Autodesk Inventor part; units mm, degrees
ref_plane "YZ Plane" through (0, 0, 0) normal (1, 0, 0) x (0, 1, 0)
ref_plane "XZ Plane" through (0, 0, 0) normal (0, 1, 0) x (-1, 0, 0)
ref_plane "XY Plane" through (0, 0, 0) normal (0, 0, 1) x (1, 0, 0)
sketch "Sketch1" plane through (0, 0, 0) normal (0, 0, 1) x (1, 0, 0)
  line L0 (-25.4, 63.5) -> (25.4, 63.5)
  line L1 (38.1, 50.8) -> (38.1, -50.8)
  line L2 (25.4, -63.5) -> (-25.4, -63.5)
  line L3 (-38.1, -50.8) -> (-38.1, 50.8)
  line L4 (-38.1, 63.5) -> (38.1, -63.5) construction
  line L5 (38.1, 63.5) -> (-38.1, -63.5) construction
  arc A0 (-25.4, 63.5) -> (-38.1, 50.8) centre (-25.4, 50.8) ccw
  arc A1 (38.1, 50.8) -> (25.4, 63.5) centre (25.4, 50.8) ccw
  arc A2 (25.4, -63.5) -> (38.1, -50.8) centre (25.4, -50.8) ccw
  arc A3 (-38.1, -50.8) -> (-25.4, -63.5) centre (-25.4, -50.8) ccw
  line L6 (25.4, 69.85) -> (-25.4, 69.85)
  arc A4 (-25.4, 69.85) -> (-44.45, 50.8) centre (-25.4, 50.8) ccw
  line L7 (-44.45, 50.8) -> (-44.45, -50.8)
  arc A5 (-44.45, -50.8) -> (-25.4, -69.85) centre (-25.4, -50.8) ccw
  line L8 (-25.4, -69.85) -> (25.4, -69.85)
  arc A6 (25.4, -69.85) -> (44.45, -50.8) centre (25.4, -50.8) ccw
  line L9 (44.45, -50.8) -> (44.45, 50.8)
  arc A7 (44.45, 50.8) -> (25.4, 69.85) centre (25.4, 50.8) ccw
  point P0 (0, 0)
  dimension "d0" = 127
  dimension "d1" = 76.2
  dimension "d2" = 12.7
  dimension "d3" = 6.35
extrude "Extrusion1" add sketch "Sketch1" against normal blind 127
properties part number "class1" material "Iron, Ductile"
Build history of the part. All positions in model axes, mm. A direction names the side the tool comes from. Round coordinates to 2 decimals unless told otherwise and drop trailing zeros. Write each loop counter-clockwise with the first axis right and the second up, starting at its lowest first coordinate (ties: lowest second). Pieces come first, ordered by that corner, then holes.
1) Drill centre lines: probe 1 along Y at (x, z) = (-15.5, -71); probe 2 along X at (y, z) = (6, -114); probe 3 along X at (y, z) = (56, -6.5). Where is each one in solid material? Low to high.
2) 3-axis set-ups, long thin cutter, end or side, ignore diameter. For faces 5 (the flat face through (0, -63.5, -63)), 6 (the flat face through (-40, 6, -127)): which of +Z, -Z, +X, -X, +Y, -Y reach the whole face in a straight line?
3) Pin check, flat tip, straight feed: pin 1 (2 mm diameter, centred on x = -35.5, z = -69, fed in from -Y). Stop position of the tip, or through.
4) Mould opens along X. For faces 1 (the flat face through (0, 69.85, -63)), 2 (the flat face through (-44.45, 1, -63)), 3 (the flat face through (38.1, 1, -63)), 4 (the cylindrical face through (39.02, 64.12, -62.61)) say: +X half, -X half, draft (parallel to the pull), parting line (faces both ways), or undercut.
5) Band-saw the part on A-A, the plane y = -48.5. List the corners of the cut face in (x, z).
6) Band-saw the part on C-C, the plane z = -106. List the corners of the cut face in (x, y), and give its area (3 significant figures).
7) Band-saw the part on B-B, the plane x = 4. List the corners of the cut face in (y, z), and give its area (3 significant figures).
Ans:
1. probe 1: y = -69.85 to -63.5, 63.5 to 69.85
1. probe 2: x = -44.45 to -38.1, 38.1 to 44.45
1. probe 3: x = -43.73 to -36.99, 36.99 to 43.73
2. face 5: +Z, -Z
2. face 6: -Z, +X, -X, +Y, -Y
3. pin 1: stops at y = -67.54
4. face 1: draft
4. face 2: -X half
4. face 3: undercut
4. face 4: +X half
5. outline: (-44.45, -127) - (-38.1, -127) - (-38.1, 0) - (-44.45, 0) - close; (38.1, -127) - (44.45, -127) - (44.45, 0) - (38.1, 0) - close
6. outline: (-44.45, -50.8) arc R19.05 ccw to (-25.4, -69.85) - (25.4, -69.85) arc R19.05 ccw to (44.45, -50.8) - (44.45, 50.8) arc R19.05 ccw to (25.4, 69.85) - (-25.4, 69.85) arc R19.05 ccw to (-44.45, 50.8) - close; hole (-38.1, -50.8) arc R12.7 ccw to (-25.4, -63.5) - (25.4, -63.5) arc R12.7 ccw to (38.1, -50.8) - (38.1, 50.8) arc R12.7 ccw to (25.4, 63.5) - (-25.4, 63.5) arc R12.7 ccw to (-38.1, 50.8) - close
6. area: 2,570 mm2
7. outline: (-69.85, -127) - (-63.5, -127) - (-63.5, 0) - (-69.85, 0) - close; (63.5, -127) - (69.85, -127) - (69.85, 0) - (63.5, 0) - close
7. area: 1,610 mm2
